Here's how the part is built. I have some questions about the finished solid (model axes, mm). A direction names the side the tool comes from. Give positions to 0.01 mm unless a question says otherwise; leave off trailing zeros. Loops run counter-clockwise (first coordinate to the right, second up) from the corner with the lowest first, then second, coordinate; pieces in that order, holes last.
Q1. Suppose I cut it at A-A (x = 0). List the corners of the cut face in (y, z) for me (3 decimals).
Q2. I need wall thicknesses on probe 1 along X at (y, z) = (-8.5, 0); probe 2 along Y at (x, z) = (5, -5); probe 3 along Z at (x, y) = (-5.5, 2). Which ranges of each line are inside material? Lowest first, please.
Q3. I'm going to push flat-ended pins straight in: P1, Ø6, axis at y = -10.5, z = -1, coming from the -X side; P2, Ø17, axis at x = 0, z = 0, coming from the -Y side; P3, Ø1.5, axis at x = -1.5, y = -11, coming from the -Z side. Where does each tip first touch, or does it pass through?
Q4. For faces 1 (the face through (-4, -4, 4)), 2 (the face through (4.84, 1.04, 15.38)), 3 (the face through (1.9, 4, 5.1)), which set-ups out of +Z, -Z, +X, -X, +Y, -Y let a thin tool reach every point of the face, with its end or its side?
Q5. Suppose I cut it at B-B (z = 0). List the corners of the cut face in (x, y) for me (3 decimals).
Q6. Suppose I cut it at C-C (y = -16.25). List the corners of the cut face in (x, z) for me, and give its area (3 significant figures).
Q7. Suppose I cut it at D-D (z = -12). List the corners of the cut face in (x, y) for me.
```python
from build123d import *

# Parameters (mm, degrees)
SKETCH1_R           = 50
BOSS_EXTRUDE1_DEPTH = 4
SKETCH2_R           = 16.125
SKETCH2_R_2         = 7.875
CUT_EXTRUDE1_DEPTH  = 6
SKETCH3_R           = 5.25
CUT_EXTRUDE2_DEPTH  = 72.161787499
SKETCH4_R           = 15.25
SKETCH4_R_2         = 10.25
BOSS_EXTRUDE2_DEPTH = 20


with BuildPart() as part:
    # Sketch1 → Boss-Extrude1 (new, symmetric)
    with BuildSketch(Plane(origin=(0, 0, 0), x_dir=(1, 0, 0), z_dir=(0, 1, 0))):
        with Locations(Location((0, 0, 0), (0, 0, 270))):
            Circle(SKETCH1_R)
    extrude(amount=BOSS_EXTRUDE1_DEPTH, both=True)

    # Sketch2 → Cut-Extrude1 (cut)
    with BuildSketch(Plane(origin=(0, 4, 0), x_dir=(1, 0, 0), z_dir=(0, 1, 0))):
        with Locations(Location((0, 0, 0), (0, 0, 270))):
            Circle(SKETCH2_R)
        with Locations(Location((0, 0, 0), (0, 0, 270))):
            Circle(SKETCH2_R_2, mode=Mode.SUBTRACT)
    extrude(amount=-CUT_EXTRUDE1_DEPTH, mode=Mode.SUBTRACT)

    # Sketch3 → Cut-Extrude2 (cut, through all)
    with BuildSketch(Plane(origin=(0, 4, 0), x_dir=(1, 0, 0), z_dir=(0, 1, 0))):
        with Locations(Location((0, 0, 0), (0, 0, 270))):
            Circle(SKETCH3_R)
    extrude(amount=-CUT_EXTRUDE2_DEPTH, mode=Mode.SUBTRACT)

    # Sketch4 → Boss-Extrude2 (add)
    with BuildSketch(Plane.XZ.offset(4)):
        with Locations(Location((0, 0, 0), (0, 0, 90))):
            Circle(SKETCH4_R)
        with Locations(Location((0, 0, 0), (0, 0, 270))):
            Circle(SKETCH4_R_2, mode=Mode.SUBTRACT)
    extrude(amount=BOSS_EXTRUDE2_DEPTH)


solid = part.part
```
Solutions:
1. outline: (-24, -15.25) - (-4, -15.25) - (-4, -50) - (4, -50) - (4, -16.125) - (-2, -16.125) - (-2, -7.875) - (4, -7.875) - (4, -5.25) - (-4, -5.25) - (-4, -10.25) - (-24, -10.25) - close; (-24, 10.25) - (-4, 10.25) - (-4, 5.25) - (4, 5.25) - (4, 7.875) - (-2, 7.875) - (-2, 16.125) - (4, 16.125) - (4, 50) - (-4, 50) - (-4, 15.25) - (-24, 15.25) - close
2. probe 1: x = -15.25 to -10.25, 10.25 to 15.25
2. probe 2: y = -4 to 4
2. probe 3: z = -49.7 to -15.16, -5.64 to 5.64, 15.16 to 49.7
3. P1: stops at x = -15.25
3. P2: stops at y = -4
3. P3: stops at z = -15.23
4. face 1: -Y
4. face 2: +Y
4. face 3: +Z, -Z, +X, -X, +Y
5. outline: (-50, -4) - (-15.25, -4) - (-15.25, -24) - (-10.25, -24) - (-10.25, -4) - (-5.25, -4) - (-5.25, 4) - (-7.875, 4) - (-7.875, -2) - (-16.125, -2) - (-16.125, 4) - (-50, 4) - close; (5.25, -4) - (10.25, -4) - (10.25, -24) - (15.25, -24) - (15.25, -4) - (50, -4) - (50, 4) - (16.125, 4) - (16.125, -2) - (7.875, -2) - (7.875, 4) - (5.25, 4) - close
6. outline: circle Ø30.5 at (0, 0); hole circle Ø20.5 at (0, 0)
6. area: 401 mm2
7. outline: (-48.54, -4) - (-9.41, -4) - (-9.41, -24) - (9.41, -24) - (9.41, -4) - (48.54, -4) - (48.54, 4) - (10.77, 4) - (10.77, -2) - (-10.77, -2) - (-10.77, 4) - (-48.54, 4) - close
